```python
from build123d import *

# Parameters (mm, degrees)
F0_R     = 6.078895
F1_DEPTH = 7.62
F2_R     = 1.778
F3_T     = -1.27


with BuildPart() as f1:
    # F0 (on Right) → F1 (new body)
    with BuildSketch(Plane.YZ):
        Circle(F0_R)
    extrude(amount=F1_DEPTH)

    # F2
    f2_edges = [f1.edges().sort_by_distance(p)[0] for p in [
        (0, -6.078895, 0),
    ]]
    fillet(f2_edges, radius=F2_R)

    # F3
    f3_openings = [f1.faces().sort_by_distance(p)[0] for p in [
        (7.62, 0, 0),
    ]]
    offset(amount=F3_T, openings=f3_openings)


solid = f1.part
```
Geometry check sheet. Reference: the model listing, model coordinates, mm. A direction names the side the tool comes from. Coordinates: 2 decimals unless noted, no trailing zeros. Order: outer loops, then holes, each group sorted by start corner. A loop starts at its lowest first (then second) coordinate and runs counter-clockwise, first axis right, second up. Notation, with made-up numbers: M 68.25,11 L 83.25,11 A23 cw 83.25,21 Z; hole C 82.5,-32 d3. An arc over 180 degrees is marked long. One line per question, with ' | ' between items. Start each with the question number.
Item 1: Material ranges on L1, parallel to Z at x = 4.1, y = 0; L2, parallel to Z at x = 4.25, y = -3; L3, parallel to Y at x = 4, z = -1.5, recorded low to high. Write a range as [from, to].
Item 2: Draft check along Z on faces 3 (the cylindrical face through (4.658, 5.798, 1.826)), 4 (the flat face through (0, 0, 0)), 5 (the flat face through (1.27, 0, 0)). Enter one of: pulls with the +Z half, pulls with the -Z half, needs draft (parallel to the pull), parting line crosses it, or undercut.
Item 3: Gauge pin test, flat ends, axial feed: pin 1 (3 mm diameter, centred on x = 5, y = -3.5, fed in from +Z); pin 2 (1.5 mm diameter, centred on x = 6, y = 4, fed in from -Z); pin 3 (2 mm diameter, centred on x = 6.5, z = -2, fed in from -Y). Record the tip position at first contact, or that the pin passes through.
Item 4: Cross-section at C-C on x = 4.5. Enter the section's corners in (y, z).
Item 5: Cross-section at A-A on z = 0. Enter the section's corners in (x, y), then the cut area to 3 significant figures.
Item 6: Set-up check for faces 1 (the flat face through (7.62, -5, -2)), 2 (the cylindrical face through (4.658, 4.442, -1.842)): record each of +Z, -Z, +X, -X, +Y, -Y from which the full face is reachable in a straight line by a thin tool's end or side.
Item 7: Cross-section at D-D on x = 0.5. Enter the section's corners in (y, z).
Findings:
1) L1: z = [-6.08, -4.81], [4.81, 6.08] | L2: z = [-5.29, -3.76], [3.76, 5.29] | L3: y = [-5.89, -4.57], [4.57, 5.89]
2) face 3: parting line crosses it | face 4: needs draft | face 5: undercut
3) pin 1: stops at z = 5.74 | pin 2: stops at z = -5.14 | pin 3: stops at y = -6
4) outline: C 0,0 d12.16; hole C 0,0 d9.62
5) outline: M 0,-4.3 A1.78 ccw 1.78,-6.08 L 7.62,-6.08 L 7.62,-4.81 L 1.78,-4.81 A0.51 cw 1.27,-4.3 L 1.27,4.3 A0.51 cw 1.78,4.81 L 7.62,4.81 L 7.62,6.08 L 1.78,6.08 A1.78 ccw 0,4.3 Z | area: 30.3 mm²
6) face 1: +Z, -Z, +X, +Y, -Y | face 2: +X
7) outline: C 0,0 d11.07
